```python
from build123d import *

# Parameters (mm, degrees)
SKETCH_1_W          = 12
SKETCH_1_H          = 23
EXTRUDE_1_DEPTH     = 26
SKETCH_2_R          = 2.332740267
EXTRUDE_2_DEPTH     = 3
SKETCH_3_W          = 1
SKETCH_3_H          = 32
EXTRUDE_3_DEPTH     = 12
SKETCH_4_R          = 1.308316264
SKETCH_4_R_2        = 1.22970194
CUT_EXTRUDE_1_DEPTH = 10


with BuildPart() as part:
    # 草图1 → 凸台-拉伸1 (new body)
    with BuildSketch(Plane.XY):
        with Locations((4.532123023, 1.863128492)):
            Rectangle(SKETCH_1_W, SKETCH_1_H)
    extrude(amount=EXTRUDE_1_DEPTH)

    # 草图2 → 凸台-拉伸2 (add)
    with BuildSketch(Plane.XY.offset(26)):
        with Locations((4.532123023, 7.613128492)):
            Circle(SKETCH_2_R)
    extrude(amount=EXTRUDE_2_DEPTH)

    # 草图3 → 凸台-拉伸3 (add)
    with BuildSketch(Plane(origin=(10.532123023, 0, 0), x_dir=(0, 0, -1), z_dir=(1, 0, 0))):
        with Locations((-20.4, 1.919988583)):
            Rectangle(SKETCH_3_W, SKETCH_3_H)
    extrude(amount=-EXTRUDE_3_DEPTH)

    # 草图4 → 切除-拉伸1 (cut)
    with BuildSketch(Plane.XY.offset(20.9)):
        with Locations((4.532123023, 15.753010852)):
            Circle(SKETCH_4_R)
        with Locations((4.532123023, -11.827886658)):
            Circle(SKETCH_4_R_2)
    extrude(amount=-CUT_EXTRUDE_1_DEPTH, mode=Mode.SUBTRACT)


solid = part.part
```
Check sheet for the modelled part. Datum: model origin and axes. Units: mm. A direction names the side the tool comes from. Coordinates: 2 decimals unless noted, no trailing zeros. Loops run counter-clockwise (first coordinate to the right, second up) from the corner with the lowest first, then second, coordinate; pieces in that order, holes last.
1) Gauge pin test, flat ends, axial feed: pin 1 (3.5 mm diameter, centred on x = 3, z = 7.5, fed in from +Y); pin 2 (4 mm diameter, centred on x = 4.53, y = 15.75, fed in from +Z); pin 3 (2 mm diameter, centred on x = 2.5, y = -12.5, fed in from -Z); pin 4 (2 mm diameter, centred on x = 4.53, y = -11.83, fed in from +Z). Record the tip position at first contact, or that the pin passes through.
2) Material ranges on probe 1 along Y at (x, z) = (9, 18); probe 2 along Z at (x, y) = (2.75, -2); probe 3 along Z at (x, y) = (7.75, -10.5), recorded low to high.
3) Sectioned sample at B-B (y = -10). Record the boundary of the cut face in (x, z), and give its area (3 significant figures).
4) Release check for a two-part mould opening along Y. For faces 4 (the face through (4, -9.637, 23)), 5 (the face through (4, 2, 26)), 6 (the face through (5.235, 16.856, 20.407)) record: released by +Y, released by -Y, zero draft, split by the parting line, or undercut.
5) Sectioned sample at C-C (x = 5). Record the boundary of the cut face in (y, z).
6) Sectioned sample at A-A (x = 1). Record the boundary of the cut face in (y, z), and give its area (3 significant figures).
7) Access from +Z, -Z, +X, -X, +Y, -Y to the whole of each face (thin tool, end or side, straight path). Record for faces 1 (the face through (4, 13.363, 23)), 2 (the face through (3, -12, 20.9)), 3 (the face through (6, 16, 19.9)).
8) Sectioned sample at D-D (z = 16.5). Record the boundary of the cut face in (x, y).
Check sheet entries:
1. pin 1: stops at y = 13.36
1. pin 2: stops at z = 20.9
1. pin 3: stops at z = 19.9
1. pin 4: passes through
2. probe 1: y = -9.64 to 13.36
2. probe 2: z = 0 to 26
2. probe 3: z = 19.9 to 20.9
3. outline: (-1.47, 19.9) - (10.53, 19.9) - (10.53, 20.9) - (-1.47, 20.9) - close
3. area: 12.0 mm2
4. face 4: released by -Y
4. face 5: zero draft
4. face 6: undercut
5. outline: (-14.08, 19.9) - (-12.97, 19.9) - (-12.97, 20.9) - (-14.08, 20.9) - close; (-10.69, 19.9) - (-9.64, 19.9) - (-9.64, 0) - (13.36, 0) - (13.36, 19.9) - (14.53, 19.9) - (14.53, 20.9) - (13.36, 20.9) - (13.36, 26) - (9.9, 26) - (9.9, 29) - (5.33, 29) - (5.33, 26) - (-9.64, 26) - (-9.64, 20.9) - (-10.69, 20.9) - close; (16.97, 19.9) - (17.92, 19.9) - (17.92, 20.9) - (16.97, 20.9) - close
6. outline: (-14.08, 19.9) - (-9.64, 19.9) - (-9.64, 0) - (13.36, 0) - (13.36, 19.9) - (17.92, 19.9) - (17.92, 20.9) - (13.36, 20.9) - (13.36, 26) - (-9.64, 26) - (-9.64, 20.9) - (-14.08, 20.9) - close
6. area: 607 mm2
7. face 1: +Z, +X, -X, +Y
7. face 2: +Z, +X, -X, -Y
7. face 3: -Z, +X, -X, +Y
8. outline: (-1.47, -9.64) - (10.53, -9.64) - (10.53, 13.36) - (-1.47, 13.36) - close
